Input: part model. Units: mm. Frame: model coordinates. A direction names the side the tool comes from. Coordinates: 2 decimals unless noted, no trailing zeros. Write each loop counter-clockwise with the first axis right and the second up, starting at its lowest first coordinate (ties: lowest second). Pieces come first, ordered by that corner, then holes. Notation, with made-up numbers: (1, -17) - (19, -17) arc R22 cw to (19, -9) - close; hole circle Ø10 at (14, 74.5). An arc over 180 degrees is marked (long way). One line per question, with ' | ' between items. Start each with the question number.
1) Reachability of faces 5 (the cylindrical face through (12.605, -8.895, 22.4)), 6 (the flat face through (10, -28, 3)), 7 (the flat face through (16, 0, 0)) from +Z, -Z, +X, -X, +Y, -Y: full face, straight path, thin tool, end or side. Return the list, or none.
2) Section query C-C on y = 0. Return loops of the section in (x, z), and give its area (3 significant figures).
3) Section query B-B on z = 0. Return loops of the section in (x, y), and give its area (3 significant figures).
4) First-contact query: P1, Ø7, axis at y = 25, z = 1.5, coming from the -X side; P2, Ø9, axis at y = 7.5, z = 4, coming from the -X side; P3, Ø2.5, axis at x = 8, y = -28, coming from the +Z side; P4, Ø3, axis at x = 4, y = -12, coming from the -Z side. Flat tips, straight axial feed; report the tip coordinate or a pass-through.
5) Section query D-D on x = 2.75. Return loops of the section in (y, z).
6) Section query A-A on x = 17.75. Return loops of the section in (y, z), and give its area (3 significant figures).
7) Line query: line 1 (Y direction, x = 3.1, z = 0); line 2 (Z direction, x = 18, y = -9); line 3 (Y direction, x = 1.75, z = -2). Output: solid intervals per line, ascending.
8) Draft query along Y for faces 1 (the flat face through (10, -28, -3)), 2 (the flat face through (10, -27, 0)), 3 (the cylindrical face through (2.54, -13.35, -16.49)), 4 (the cylindrical face through (9.86, 5.267, 29.534)). Return one class per face: released by +Y, released by -Y, zero draft, split by the parting line, or undercut.
Autodesk Inventor part; units mm, degrees
ref_plane "РабПлоскость1" through (10, -29.8496, -3) normal (-1, 0, 0) x (0, 0, 1)
ref_plane "YZ Plane" through (0, 0, 0) normal (1, 0, 0) x (0, 1, 0)
ref_plane "XZ Plane" through (0, 0, 0) normal (0, 1, 0) x (-1, 0, 0)
sketch "Эскиз1" plane through (0, 0, 0) normal (0, 0, 1) x (1, 0, 0)
  line L0 (0, 0) -> (20, 0)
  line L1 (20, 0) -> (20, 30)
  line L2 (20, 30) -> (0, 30)
  line L3 (0, 30) -> (0, 0)
  dimension "d0" = 20
  dimension "d1" = 30
revolve "Вращение1" add sketch "Эскиз1" angle 360 about axis through (0, 0, 0) along (1, 0, 0)
sketch "Эскиз2" plane through (0, 0, 0) normal (-1, 0, 0) x (0, 0, 1)
  point P0 (0, 0)
  point P1 (0, 24)
  point P2 (-20.7846, -12)
  point P3 (20.7846, -12)
  dimension "d3" = 24
  dimension "d6" = 360
hole "Отверстие1" at (0, 24, 0) at (0, -12, -20.7846) at (0, -12, 20.7846) direction (1, 0, 0) diameter 7 end through all counterbore diameter 9 counterbore depth 5
sketch "Эскиз3" plane through (0, 0, 0) normal (-1, 0, 0) x (0, 0, 1)
  point P0 (0, 0)
  point P1 (0, 0)
hole "Отверстие2" at (0, 0, 0) direction (1, 0, 0) diameter 30 depth 16 countersink diameter 34 countersink angle 90
sketch "Эскиз4" plane through (0, 0, 0) normal (-1, 0, 0) x (0, 0, 1)
  circle A0 centre (0, 0) radius 30 construction
  line L0 (-3, -27) -> (3, -27)
  line L1 (3, -27) -> (3, -29.8496)
  line L2 (-3, -29.8496) -> (-3, -27)
  arc A1 (-3, -29.8496) -> (3, -29.8496) centre (0, 0) ccw
  point P0 (0, -27)
  dimension "d22" = 6
  dimension "d23" = 27
extrude "Выдавливание1" cut sketch "Эскиз4" against normal blind 20
ref_plane "РабПлоскость1" through (10, -29.8496, -3) normal (-1, 0, 0) x (0, 0, 1)
sketch "Эскиз5" plane through (10, -29.8496, -3) normal (-1, 0, 0) x (0, 0, 1)
  line L0 (3, 29.8496) -> (-21.7487, 54.5984) construction
  line L1 (3, 29.8496) -> (33, 29.8496) construction
  arc A0 (6, 0) -> (0, 0) centre (3, 29.8496) ccw construction
  circle A1 centre (3, 29.8496) radius 15 construction
  arc A2 (-6.0161, 41.8375) -> (-8.9879, 38.8657) centre (3, 29.8496) ccw
  line L2 (-7.6066, 40.4562) -> (-21.7487, 54.5984)
  line L3 (-6.0161, 41.8375) -> (-16.4454, 59.9017)
  line L4 (-8.9879, 38.8657) -> (-27.052, 49.2951)
  line L5 (-27.052, 49.2951) -> (-16.4454, 59.9017)
  dimension "d27" = 135
  dimension "d32" = 15
  dimension "d33" = 15
  dimension "d34" = 20
  dimension "d35" = 15
revolve "Вращение3" cut sketch "Эскиз5" angle 360 about axis through (10, 0, 0) along (0, 0.7071068, -0.7071068) contours A2 L2 L5 L3
properties part number "711124"
Answer key:
1) face 5: +X, -X | face 6: +X, -X, -Y | face 7: -X
2) outline: (0, -30) - (20, -30) - (20, 30) - (0, 30) - (0, 17) - (2, 15) - (16, 15) - (16, -15) - (2, -15) - (0, -17) - close | area: 716 mm²
3) outline: (0, -27) - (20, -27) - (20, 20.5) - (5, 20.5) - (5, 19.5) - (0, 19.5) - (0, 17) - (2, 15) - (16, 15) - (16, -15) - (2, -15) - (0, -17) - close; (0, 28.5) - (5, 28.5) - (5, 27.5) - (20, 27.5) - (20, 30) - (0, 30) - close | area: 506 mm²
4) P1: x = 0 | P2: x = 16 | P3: z = 13.58 | P4: z = -28.1
5) outline: (-29.85, -3) arc R30 ccw (long way) to (-29.85, 3) - (-27, 3) - (-27, -3) - close; hole circle Ø9 at (-12, -20.78); hole circle Ø9 at (-12, 20.78); hole circle Ø30 at (0, 0); hole circle Ø9 at (24, 0)
6) outline: (-29.85, -3) arc R30 ccw (long way) to (-29.85, 3) - (-27, 3) - (-27, -3) - close; hole circle Ø7 at (-12, -20.78); hole circle Ø7 at (-12, 20.78); hole circle Ø7 at (24, 0) | area: 2,690 mm²
7) line 1: -27 to -15, 15 to 19.5, 28.5 to 30 | line 2: -28.62 to -22.59, -18.98 to 18.98, 22.59 to 28.62 | line 3: -27 to -15.12, 15.12 to 19.97, 28.03 to 29.93
8) face 1: zero draft | face 2: released by -Y | face 3: undercut | face 4: split by the parting line
